Geometry check sheet. Reference: drawing and pictorial views, mm from the part's lowest x, y, z. A direction names the side the tool comes from. Round coordinates to 2 decimals unless told otherwise and drop trailing zeros. Order: outer loops, then holes, each group sorted by start corner. A loop starts at its lowest first (then second) coordinate and runs counter-clockwise, first axis right, second up.
(1) Sectioned sample at A-A (z = 1). Record the boundary of the cut face in (x, y) (1 decimal), plus the area to 3 significant figures.
(2) Set-up check for the marked faces 1 and 2: record each of +Z, -Z, +X, -X, +Y, -Y from which the full face is reachable in a straight line by a thin tool's end or side.
(3) Sectioned sample at D-D (x = 52). Record the boundary of the cut face in (y, z), plus the area to 3 significant figures.
(4) Sectioned sample at C-C (x = 28). Record the boundary of the cut face in (y, z).
(5) Material ranges on line 1 along X through (y, z) = (31.5, 3) (1 decimal); line 2 along Y through (x, z) = (23, 1.8); line 3 along X through (y, z) = (37, 2.2) (1 decimal), recorded low to high.
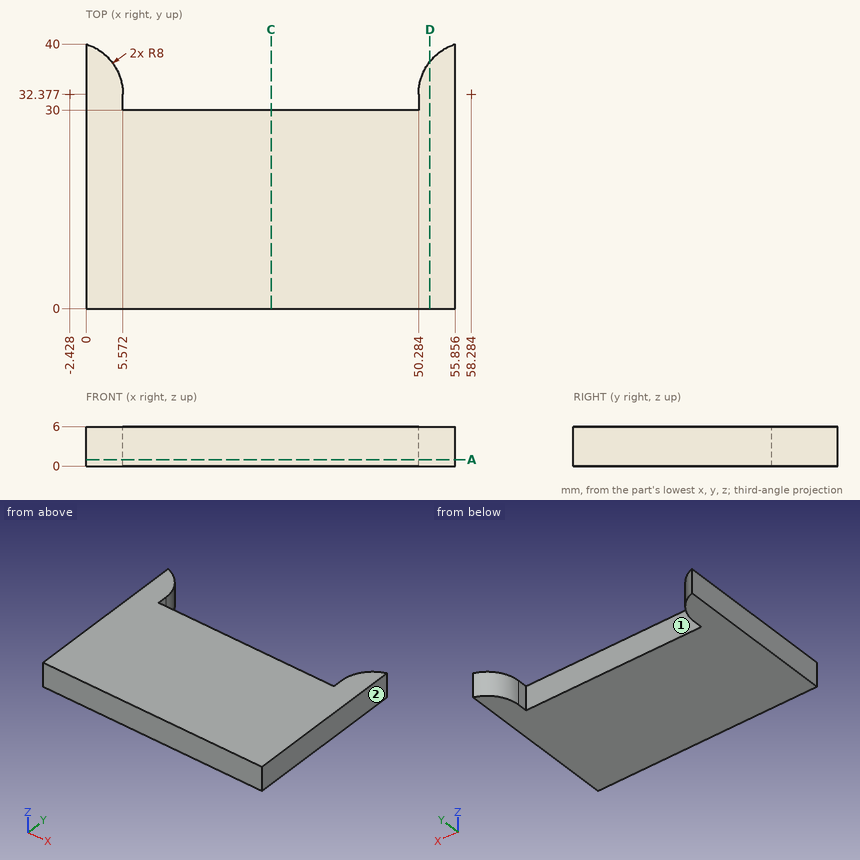
Answer below:
1. outline: (0, 0) - (55.9, 0) - (55.9, 40) arc R8 ccw to (50.3, 32.4) - (50.3, 30) - (5.6, 30) - (5.6, 32.4) arc R8 ccw to (0, 40) - close
1. area: 1,760 mm2
2. face 1: +Z, -Z, +Y
2. face 2: +Z, -Z, +X, +Y, -Y
3. outline: (0, 0) - (37.33, 0) - (37.33, 6) - (0, 6) - close
3. area: 224 mm2
4. outline: (0, 0) - (30, 0) - (30, 6) - (0, 6) - close
5. line 1: x = 0 to 5.6, 50.3 to 55.9
5. line 2: y = 0 to 30
5. line 3: x = 0 to 4.1, 51.8 to 55.9
